Source: CAD feature listing. Evaluate the final solid. Frame: model axes, mm. A direction names the side the tool comes from. Give positions to 0.01 mm unless a question says otherwise; leave off trailing zeros. Write each loop counter-clockwise with the first axis right and the second up, starting at its lowest first coordinate (ties: lowest second). Pieces come first, ordered by that corner, then holes. Notation, with made-up numbers: (78, 11.25) - (104, 11.25) arc R15 ccw to (104, 36.25) - close; hole circle Ø7 at (86, 68). An arc over 180 degrees is marked (long way). One line per question, with ' | ' between items. Start each with the question number.
(1) Ray query, line 1 (Y direction, x = 0.75, z = 0.5); line 2 (X direction, y = -5.5, z = -0.1); line 3 (Z direction, x = 0.15, y = -4.5). Return the intervals inside material, ascending. Write a range as [from, to].
(2) Section A-A, the plane x = 0. Return loops of the section in (y, z) (3 decimals).
(3) Section C-C, the plane y = 4.5. Return loops of the section in (x, z) (3 decimals).
(4) Access query for faces 1 (the flat face through (-1, 0, 0)), 2 (the flat face through (0, 1, 1.27)). Directions: +Z, -Z, +X, -X, +Y, -Y. A direction counts if a zero-diameter tool reaches every point of the face in a straight line with its end or side. Return the directions, or none.
(5) Section D-D, the plane x = 0.9. Return loops of the section in (y, z), plus the area to 3 significant figures.
(6) Section B-B, the plane z = 0. Return loops of the section in (x, y) (3 decimals), plus the area to 3 significant figures.
(7) Draft query along X for faces 3 (the flat face through (-1, 2.5, 0)), 4 (the flat face through (-1.27, 1, 0)), 5 (the flat face through (1.27, 1, 0)). Return one class per face: +X half, -X half, draft (parallel to the pull), parting line (faces both ways), or undercut.
(8) Pin query (flat end, axial travel): pin 1 (1.3 mm diameter, centred on x = -0.5, z = 0.5, fed in from -Y). Return the tip coordinate at first contact, or that it passes through.
Autodesk Inventor part; units mm, degrees
ref_plane "YZ Plane" through (0, 0, 0) normal (1, 0, 0) x (0, 1, 0)
ref_plane "XZ Plane" through (0, 0, 0) normal (0, 1, 0) x (-1, 0, 0)
ref_plane "XY Plane" through (0, 0, 0) normal (0, 0, 1) x (1, 0, 0)
sketch "Sketch1" plane through (0, 0, 0) normal (0, 1, 0) x (-1, 0, 0)
  line L0 (-1.27, -1.27) -> (1.27, -1.27)
  line L1 (1.27, -1.27) -> (1.27, 1.27)
  line L2 (1.27, 1.27) -> (-1.27, 1.27)
  line L3 (-1.27, 1.27) -> (-1.27, -1.27)
  line L4 (-1.27, -1.27) -> (1.27, 1.27) construction
  line L5 (1.27, -1.27) -> (-1.27, 1.27) construction
  point P0 (0, 0)
  dimension "d0" = 2.54
  dimension "d1" = 2.54
extrude "Extrusion1" add sketch "Sketch1" along normal blind 2.5
sketch "Sketch2" plane through (0, 2.5, 0) normal (0, 1, 0) x (1, 0, 0)
  circle A0 centre (0, 0) radius 0.325
  dimension "d4" = 0.65
extrude "Extrusion2" add sketch "Sketch2" along normal blind 3
sketch "Sketch3" plane through (0, 0, 0) normal (0, -1, 0) x (1, 0, 0)
  circle A0 centre (0, 0) radius 0.325
  dimension "d7" = 0.65
extrude "Extrusion3" add sketch "Sketch3" along normal blind 6
properties part number "pin-header-male" material "Aluminum"
Check sheet entries:
1) line 1: [0, 2.5] | line 2: [-0.31, 0.31] | line 3: [-0.29, 0.29]
2) outline: (-6, -0.325) - (0, -0.325) - (0, -1.27) - (2.5, -1.27) - (2.5, -0.325) - (5.5, -0.325) - (5.5, 0.325) - (2.5, 0.325) - (2.5, 1.27) - (0, 1.27) - (0, 0.325) - (-6, 0.325) - close
3) outline: circle Ø0.65 at (0, 0)
4) face 1: -Y | face 2: +Z, +X, -X, +Y, -Y
5) outline: (0, -1.27) - (2.5, -1.27) - (2.5, 1.27) - (0, 1.27) - close | area: 6.35 mm²
6) outline: (-1.27, 0) - (-0.325, 0) - (-0.325, -6) - (0.325, -6) - (0.325, 0) - (1.27, 0) - (1.27, 2.5) - (0.325, 2.5) - (0.325, 5.5) - (-0.325, 5.5) - (-0.325, 2.5) - (-1.27, 2.5) - close | area: 12.2 mm²
7) face 3: draft | face 4: -X half | face 5: +X half
8) pin 1: y = -6
